Geometry check sheet. Reference: the model listing, model coordinates, mm. Face numbers are marked on the shaded views. A direction names the side the tool comes from. Coordinates: 2 decimals unless noted, no trailing zeros. Write each loop counter-clockwise with the first axis right and the second up, starting at its lowest first coordinate (ties: lowest second). Pieces come first, ordered by that corner, then holes. Notation, with made-up numbers: (30.5, 58) -> (36.5, 58) arc R14 ccw to (36.5, 69) -> close; hole circle Ø3 at (12, 25). An arc over 180 degrees is marked (long way). Answer as CSV lines item,"result".
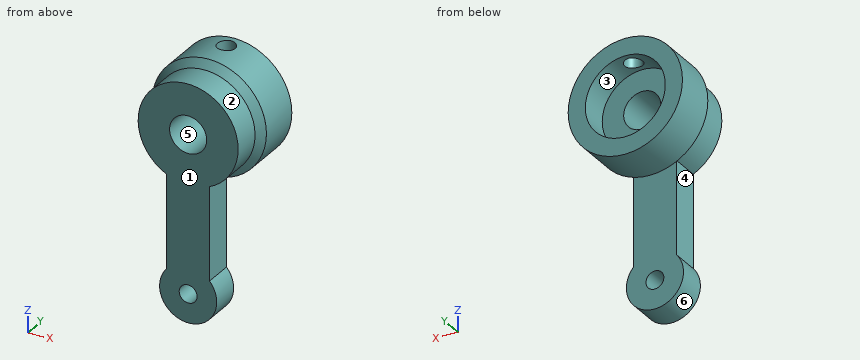
```python
from build123d import *

# Parameters (mm, degrees)
CYLINDER968_R          = 1.25
CYLINDER968_DEPTH      = 4
CYLINDER968_ROLL_ANGLE = 90
CYLINDER972_R          = 1.25
CYLINDER972_DEPTH      = 7
CYLINDER970_R          = 2.6
CYLINDER970_DEPTH      = 11
CYLINDER970_ROLL_ANGLE = 90
CYLINDER969_R          = 5.6
CYLINDER969_DEPTH      = 4
CYLINDER969_ROLL_ANGLE = 90
CYLINDER971_R          = 8
CYLINDER971_DEPTH      = 6
CYLINDER971_ROLL_ANGLE = 90
CYLINDER964_R          = 7
CYLINDER964_DEPTH      = 6
CYLINDER964_ROLL_ANGLE = 90
CYLINDER965_R          = 4
CYLINDER965_DEPTH      = 4
CYLINDER965_ROLL_ANGLE = 90
BOX564_W               = 6
BOX564_H               = 4
BOX564_DEPTH           = 22
CHAMFER105_SIZE        = 0.999


with BuildPart() as cylinder1140:
    # Cylinder968 → Cylinder968 (new body)
    with BuildSketch(Plane.XY):
        Circle(CYLINDER968_R)
    extrude(amount=CYLINDER968_DEPTH)


with BuildPart() as cylinder1140_1:
    # Cylinder968 roll: moved
    add(cylinder1140.part.rotate(Axis((0, 0, 0), (1, 0, 0)), CYLINDER968_ROLL_ANGLE))


with BuildPart() as cylinder1140_2:
    # Cylinder968 placement: moved
    add(cylinder1140_1.part.moved(Location((37, 32.75, -33))))


with BuildPart() as cylinder1144:
    # Cylinder972 → Cylinder972 (new body)
    with BuildSketch(Plane(origin=(37, 37.75, -8), x_dir=(1, 0, 0), z_dir=(0, 0, 1))):
        Circle(CYLINDER972_R)
    extrude(amount=CYLINDER972_DEPTH)


with BuildPart() as cylinder1142:
    # Cylinder970 → Cylinder970 (new body)
    with BuildSketch(Plane.XY):
        Circle(CYLINDER970_R)
    extrude(amount=CYLINDER970_DEPTH)


with BuildPart() as cylinder1142_1:
    # Cylinder970 roll: moved
    add(cylinder1142.part.rotate(Axis((0, 0, 0), (1, 0, 0)), CYLINDER970_ROLL_ANGLE))


with BuildPart() as cylinder1142_2:
    # Cylinder970 placement: moved
    add(cylinder1142_1.part.moved(Location((37, 39.75, -11))))


with BuildPart() as fusion607:
    # Cylinder969 → Cylinder969 (new body)
    with BuildSketch(Plane.XY):
        Circle(CYLINDER969_R)
    extrude(amount=CYLINDER969_DEPTH)


with BuildPart() as fusion607_1:
    # Cylinder969 roll: moved
    add(fusion607.part.rotate(Axis((0, 0, 0), (1, 0, 0)), CYLINDER969_ROLL_ANGLE))


with BuildPart() as fusion607_2:
    # Cylinder969 placement: moved
    add(fusion607_1.part.moved(Location((37, 39.75, -11))))

    # Fusion607: union Cylinder1140, Cylinder1144, Cylinder1142
    add(cylinder1140_2.part)
    add(cylinder1144.part)
    add(cylinder1142_2.part)


with BuildPart() as cylinder1143:
    # Cylinder971 → Cylinder971 (new body)
    with BuildSketch(Plane.XY):
        Circle(CYLINDER971_R)
    extrude(amount=CYLINDER971_DEPTH)


with BuildPart() as cylinder1143_1:
    # Cylinder971 roll: moved
    add(cylinder1143.part.rotate(Axis((0, 0, 0), (1, 0, 0)), CYLINDER971_ROLL_ANGLE))


with BuildPart() as cylinder1143_2:
    # Cylinder971 placement: moved
    add(cylinder1143_1.part.moved(Location((37, 39.75, -11))))


with BuildPart() as cylinder1136:
    # Cylinder964 → Cylinder964 (new body)
    with BuildSketch(Plane.XY):
        Circle(CYLINDER964_R)
    extrude(amount=CYLINDER964_DEPTH)


with BuildPart() as cylinder1136_1:
    # Cylinder964 roll: moved
    add(cylinder1136.part.rotate(Axis((0, 0, 0), (1, 0, 0)), CYLINDER964_ROLL_ANGLE))


with BuildPart() as cylinder1136_2:
    # Cylinder964 placement: moved
    add(cylinder1136_1.part.moved(Location((37, 39.75, -11))))


with BuildPart() as cylinder1137:
    # Cylinder965 → Cylinder965 (new body)
    with BuildSketch(Plane.XY):
        Circle(CYLINDER965_R)
    extrude(amount=CYLINDER965_DEPTH)


with BuildPart() as cylinder1137_1:
    # Cylinder965 roll: moved
    add(cylinder1137.part.rotate(Axis((0, 0, 0), (1, 0, 0)), CYLINDER965_ROLL_ANGLE))


with BuildPart() as cylinder1137_2:
    # Cylinder965 placement: moved
    add(cylinder1137_1.part.moved(Location((37, 37.75, -33))))


with BuildPart() as front_axle_steering_arm:
    # Box564 → Box564 (new body)
    with BuildSketch(Plane(origin=(34, 33.75, -33), x_dir=(1, 0, 0), z_dir=(0, 0, 1))):
        with Locations((3, 2)):
            Rectangle(BOX564_W, BOX564_H)
    extrude(amount=BOX564_DEPTH)

    # Fusion608: union Cylinder1136, Cylinder1137
    add(cylinder1136_2.part)
    add(cylinder1137_2.part)


with BuildPart() as front_axle_steering_arm_1:
    # Fusion608 placement: moved
    add(front_axle_steering_arm.part.moved(Location((0, -5, 0))))

    # Fusion609: union Cylinder1143
    add(cylinder1143_2.part)

    # Cut703: cut Fusion607
    add(fusion607_2.part, mode=Mode.SUBTRACT)

    # Chamfer105
    chamfer105_edges = [front_axle_steering_arm_1.edges().sort_by_distance(p)[0] for p in [
        (30, 33.75, -11),
    ]]
    chamfer(chamfer105_edges, length=CHAMFER105_SIZE)


solid = front_axle_steering_arm_1.part
```
Item 1: Depth check by flat-ended pin: pin 1 Ø3 at (y, z) = (30, -30.5) entering from +X; pin 2 Ø4.5 at (y, z) = (31, -21.5) entering from -X; pin 3 Ø2 at (x, y) = (35, 31.5) entering from -Z; pin 4 Ø1.5 at (x, z) = (37, -33) entering from -Y. Enter the tip coordinate at first touch or a pass-through.
Responses:
pin 1,"stops at x = 40.87"
pin 2,"stops at x = 34"
pin 3,"stops at z = -36.87"
pin 4,"passes through"
Item 2: Release check for a two-part mould opening along X. For the marked faces 4, 5 and 6 record: +X half, -X half, draft (parallel to the pull), parting line (faces both ways), or undercut.
Responses:
face 4,"-X half"
face 5,"undercut"
face 6,"parting line"
Item 3: Cross-section at B-B, the plane x = 37. Count the separate pieces of the cut face and the enclosed holes in it, plus the area to 3 significant figures.
Responses:
separate pieces,"4"
enclosed holes,"0"
area,"146 mm2"
Item 4: Cross-section at C-C, the plane y = 30. Record the cut outline in (x, z), plus the area to 3 significant figures.
Responses:
outline,"(34, -30.35) arc R4 ccw (long way) to (40, -30.35) -> (40, -17.32) arc R7 ccw (long way) to (34, -17.32) -> close; hole circle Ø5.2 at (37, -11); hole circle Ø2.5 at (37, -33)"
area,"248 mm2"
Item 5: Thickness scan on probe 1 along Z at (x, y) = (37, 31.7); probe 2 along X at (y, z) = (30.15, -33); probe 3 along Z at (x, y) = (37.75, 29.5). Record the ranges inside material, lowest first.
Responses:
probe 1,"z = -37 to -34.25, -31.75 to -13.6, -8.4 to -4"
probe 2,"x = 33 to 35.75, 38.25 to 41"
probe 3,"z = -36.93 to -34, -32 to -13.49, -8.51 to -4.04"
Item 6: Cross-section at A-A, the plane z = -33. Record the cut outline in (x, y), plus the area to 3 significant figures.
Responses:
outline,"(33, 28.75) -> (35.75, 28.75) -> (35.75, 32.75) -> (33, 32.75) -> close; (38.25, 28.75) -> (41, 28.75) -> (41, 32.75) -> (38.25, 32.75) -> close"
area,"22.0 mm2"
Item 7: Set-up check for the marked faces 1, 2 and 3: record each of +Z, -Z, +X, -X, +Y, -Y from which the full face is reachable in a straight line by a thin tool's end or side.
Responses:
face 1,"+Z, -Z, +X, -X, -Y"
face 2,"-Y"
face 3,"+Y"
